```python
from build123d import *

# Parameters (mm, degrees)
SKETCH10_W          = 35
SKETCH10_H          = 26
BOSS_EXTRUDE4_DEPTH = 2.5
SKETCH1_R           = 1.5
BOSS_EXTRUDE5_DEPTH = 5
SKETCH11_W          = 35
SKETCH11_H          = 26
BOSS_EXTRUDE6_DEPTH = 2.5
CUT_EXTRUDE1_START  = -13
CUT_EXTRUDE1_DEPTH  = 56.676105727
SKETCH4_R           = 7.6
CUT_EXTRUDE2_DEPTH  = 1.2
SKETCH5_R           = 6.6
CUT_EXTRUDE3_DEPTH  = 50.27874954
SKETCH8_R           = 4
CUT_EXTRUDE6_DEPTH  = 50.27874954
SKETCH13_R          = 1.5
BOSS_EXTRUDE7_DEPTH = 10
FILLET1_R           = 13
CUT_EXTRUDE11_DEPTH = 154.613950883
FILLET2_R           = 13


with BuildPart() as part:
    # Sketch10 → Boss-Extrude4 (new body)
    with BuildSketch(Plane(origin=(0, 0, 0), x_dir=(1, 0, 0), z_dir=(0, 1, 0))):
        with Locations((15.5, -23)):
            Rectangle(SKETCH10_W, SKETCH10_H)
    extrude(amount=BOSS_EXTRUDE4_DEPTH)

    # Sketch1 → Boss-Extrude5 (add)
    with BuildSketch(Plane(origin=(0, 0, 0), x_dir=(1, 0, 0), z_dir=(0, 1, 0))):
        Polygon((0, 0), (6, 0), (6, -10), (25, -10), (25, 0), (31, 0), (31, -10), (33, -10), (33, -36), (-2, -36), (-2, -10), (0, -10), align=None)
        with Locations(Location((3, -5, 0), (0, 0, 270))):
            Circle(SKETCH1_R, mode=Mode.SUBTRACT)
        with Locations(Location((28, -5, 0), (0, 0, 90))):
            Circle(SKETCH1_R, mode=Mode.SUBTRACT)
    extrude(amount=-BOSS_EXTRUDE5_DEPTH)

    # Sketch11 → Boss-Extrude6 (add)
    with BuildSketch(Plane.XZ.offset(5)):
        with Locations((15.5, 23)):
            Rectangle(SKETCH11_W, SKETCH11_H)
    extrude(amount=BOSS_EXTRUDE6_DEPTH)

    # Sketch3 → Cut-Extrude1 (cut)
    with BuildSketch(Plane(origin=(0, 0, 10), x_dir=(-1, 0, 0), z_dir=(0, 0, -1)).offset(CUT_EXTRUDE1_START)):
        Polygon((-22.1, 2.5), (-22.1, 0.2875), (-23.1, 0.2875), (-23.1, -0.9125), (-15.5, -0.9125), (-7.9, -0.9125), (-7.9, 0.2875), (-8.9, 0.2875), (-8.9, 2.5), align=None)
    cut_extrude1 = extrude(amount=CUT_EXTRUDE1_DEPTH, mode=Mode.SUBTRACT)

    # Sketch4 → Cut-Extrude2 (cut)
    with BuildSketch(Plane(origin=(0, -0.9125, 0), x_dir=(1, 0, 0), z_dir=(0, 1, 0))):
        with Locations((15.5, -23)):
            Circle(SKETCH4_R)
    cut_extrude2 = extrude(amount=CUT_EXTRUDE2_DEPTH, mode=Mode.SUBTRACT)

    # Sketch5 → Cut-Extrude3 (cut, through all)
    with BuildSketch(Plane(origin=(0, -0.9125, 0), x_dir=(1, 0, 0), z_dir=(0, 1, 0))):
        with Locations((15.5, -23)):
            Circle(SKETCH5_R)
    cut_extrude3 = extrude(amount=CUT_EXTRUDE3_DEPTH, mode=Mode.SUBTRACT)

    # Sketch8 → Cut-Extrude6 (cut, through all)
    with BuildSketch(Plane(origin=(0, -0.9125, 0), x_dir=(1, 0, 0), z_dir=(0, 1, 0))):
        with Locations(Location((15.5, -23, 0), (0, 0, 270))):
            Circle(SKETCH8_R)
    extrude(amount=-CUT_EXTRUDE6_DEPTH, mode=Mode.SUBTRACT)

    # Mirror1: Cut-Extrude1, Cut-Extrude2, Cut-Extrude3 across plane
    add(cut_extrude1.mirror(Plane.ZX.offset(-2.5)), mode=Mode.SUBTRACT)
    add(cut_extrude2.mirror(Plane.ZX.offset(-2.5)), mode=Mode.SUBTRACT)
    add(cut_extrude3.mirror(Plane.ZX.offset(-2.5)), mode=Mode.SUBTRACT)

    # Sketch13 → Boss-Extrude7 (add)
    with BuildSketch(Plane(origin=(0, 2.5, 0), x_dir=(1, 0, 0), z_dir=(0, 1, 0))):
        Polygon((-2, -36), (70.668567607, -122.603026514), (104.009911505, -94.626317146), (33, -10), (33, -36), align=None)
        with Locations(Location((51.004955752, -65.313158573, 0), (0, 0, 270))):
            Circle(SKETCH13_R, mode=Mode.SUBTRACT)
    extrude(amount=-BOSS_EXTRUDE7_DEPTH)

    # Fillet1
    fillet1_edges = [part.edges().sort_by_distance(p)[0] for p in [
        (104.009911505, -2.5, 94.626317146),
        (70.668567607, -2.5, 122.603026514),
        (-2, -2.5, 36),
    ]]
    fillet(fillet1_edges, radius=FILLET1_R)

    # Sketch18 → Cut-Extrude11 (cut, through all)
    with BuildSketch(Plane(origin=(0, 2.5, 0), x_dir=(1, 0, 0), z_dir=(0, 1, 0))):
        with BuildLine():
            Line((47.190035997, -94.622402119), (80.531379895, -66.645692751))
            Line((80.531379895, -66.645692751), (95.653672579, -84.667739385))
            ThreePointArc((95.653672579, -84.667739385), (98.645625894, -94.157002967), (94.051333744, -102.982556072))
            Line((94.051333744, -102.982556072), (80.627145367, -114.246787588))
            ThreePointArc((80.627145367, -114.246787588), (71.137881786, -117.238740903), (62.312328681, -112.644448753))
            Line((62.312328681, -112.644448753), (47.190035997, -94.622402119))
        make_face()
    extrude(amount=-CUT_EXTRUDE11_DEPTH, mode=Mode.SUBTRACT)

    # Fillet2
    fillet2_edges = [part.edges().sort_by_distance(p)[0] for p in [
        (47.190035997, -2.5, 94.622402119),
        (80.531379895, -2.5, 66.645692751),
    ]]
    fillet(fillet2_edges, radius=FILLET2_R)


solid = part.part
```
Check sheet for the modelled part. Datum: model origin and axes. Units: mm. A direction names the side the tool comes from. Coordinates: 2 decimals unless noted, no trailing zeros. Order: outer loops, then holes, each group sorted by start corner. A loop starts at its lowest first (then second) coordinate and runs counter-clockwise, first axis right, second up. Notation, with made-up numbers: M -38,-27.5 L 17,-27.5 A8 cw 17,-15.5 Z; hole C 16,33 d11. An arc over 180 degrees is marked long. One line per question, with ' | ' between items. Start each with the question number.
Item 1: Sectioned sample at B-B on x = 15.5. Record the cut outline in (y, z).
Item 2: Material ranges on line 1 (X direction, y = -3.2, z = 5); line 2 (Y direction, x = 16, z = 11.5); line 3 (Z direction, x = 28, y = -1.55), recorded low to high.
Item 3: Access from +Z, -Z, +X, -X, +Y, -Y to the whole of each face (thin tool, end or side, straight path). Record for faces 4 (the flat face through (4.4, 0, 6)), 5 (the flat face through (25, -2, 5)), 6 (the flat face through (22.1, 1, 17)), 7 (the flat face through (8.7, 0.288, 21.1)).
Item 4: Mould release check, pull along X, two halves, no side actions. Record for faces 1 (the flat face through (31, -2, 5)), 2 (the flat face through (22.1, -6, 17)), 3 (the flat face through (26.7, -5, 3.8)): pulls with the +X half, pulls with the -X half, needs draft (parallel to the pull), parting line crosses it, or undercut.
Item 5: Sectioned sample at A-A on z = 24. Record the cut outline in (x, y), and give its area (3 significant figures).
Item 6: Sectioned sample at C-C on y = -3. Record the cut outline in (x, z), and give its area (3 significant figures).
Item 7: Gauge pin test, flat ends, axial feed: P1, Ø0.6, axis at y = -4.5, z = 17.5, coming from the +X side (3 decimals); P2, Ø0.7, axis at y = 1.5, z = 17, coming from the +X side; P3, Ø5.5, axis at y = -3.5, z = 3.5, coming from the -X side. Record the tip position at first contact, or that the pin passes through.
Item 8: Sectioned sample at D-D on x = 3. Record the cut outline in (y, z).
Answer below:
1) outline: M -7.5,29.6 L -5.29,29.6 L -5.29,30.6 L -4.09,30.6 L -4.09,27 L -0.91,27 L -0.91,30.6 L 0.29,30.6 L 0.29,29.6 L 2.5,29.6 L 2.5,56.86 L -7.5,56.86 Z; M -4.09,10 L -0.91,10 L -0.91,19 L -4.09,19 Z
2) line 1: x = 0 to 1.5, 4.5 to 6, 25 to 26.5, 29.5 to 31 | line 2: y = -4.09 to -0.91 | line 3: z = 0 to 3.5, 6.5 to 71.75
3) face 4: -Z, +X, -X, +Y | face 5: -Z, +Y, -Y | face 6: -Z, +Y | face 7: -Z
4) face 1: pulls with the +X half | face 2: undercut | face 3: needs draft
5) outline: M -2,-7.5 L 8.98,-7.5 L 8.98,-5.29 L 7.97,-5.29 L 7.97,-4.09 L 11.63,-4.09 L 11.63,-0.91 L 7.97,-0.91 L 7.97,0.29 L 8.98,0.29 L 8.98,2.5 L -2,2.5 Z; M 19.37,-4.09 L 23.03,-4.09 L 23.03,-5.29 L 22.02,-5.29 L 22.02,-7.5 L 44.75,-7.5 L 44.75,2.5 L 22.02,2.5 L 22.02,0.29 L 23.03,0.29 L 23.03,-0.91 L 19.37,-0.91 Z | area: 349 mm^2
6) outline: M -2,10 L 0,10 L 0,0 L 6,0 L 6,10 L 25,10 L 25,0 L 31,0 L 31,10 L 33,10 L 72.18,56.69 A13 ccw 70.57,75 L 57.15,86.27 A13 ccw 38.83,84.66 L 1.04,39.62 A13 ccw -2,31.27 Z; hole C 3,5 d3; hole C 15.5,23 d8; hole C 28,5 d3; hole C 51,65.31 d3 | area: 3,700 mm^2
7) P1: stops at x = 39.545 | P2: stops at x = 39.17 | P3: stops at x = 0
8) outline: M -7.5,10 L -5,10 L -5,6.5 L 0,6.5 L 0,10 L 2.5,10 L 2.5,41.96 L -7.5,41.96 Z; M -5,0 L 0,0 L 0,3.5 L -5,3.5 Z
